Verification items for this drawing (mm, ordinates from the low corner). A direction names the side the tool comes from. Coordinates: 2 decimals unless noted, no trailing zeros. Order: outer loops, then holes, each group sorted by start corner. A loop starts at its lowest first (then second) coordinate and runs counter-clockwise, first axis right, second up. Notation, with made-up numbers: M 46,-6.75 L 80,-6.75 A14 cw 80,19.25 Z; hole C 51,78.25 d7. An arc over 180 degrees is marked long. Write item = value, one per line.
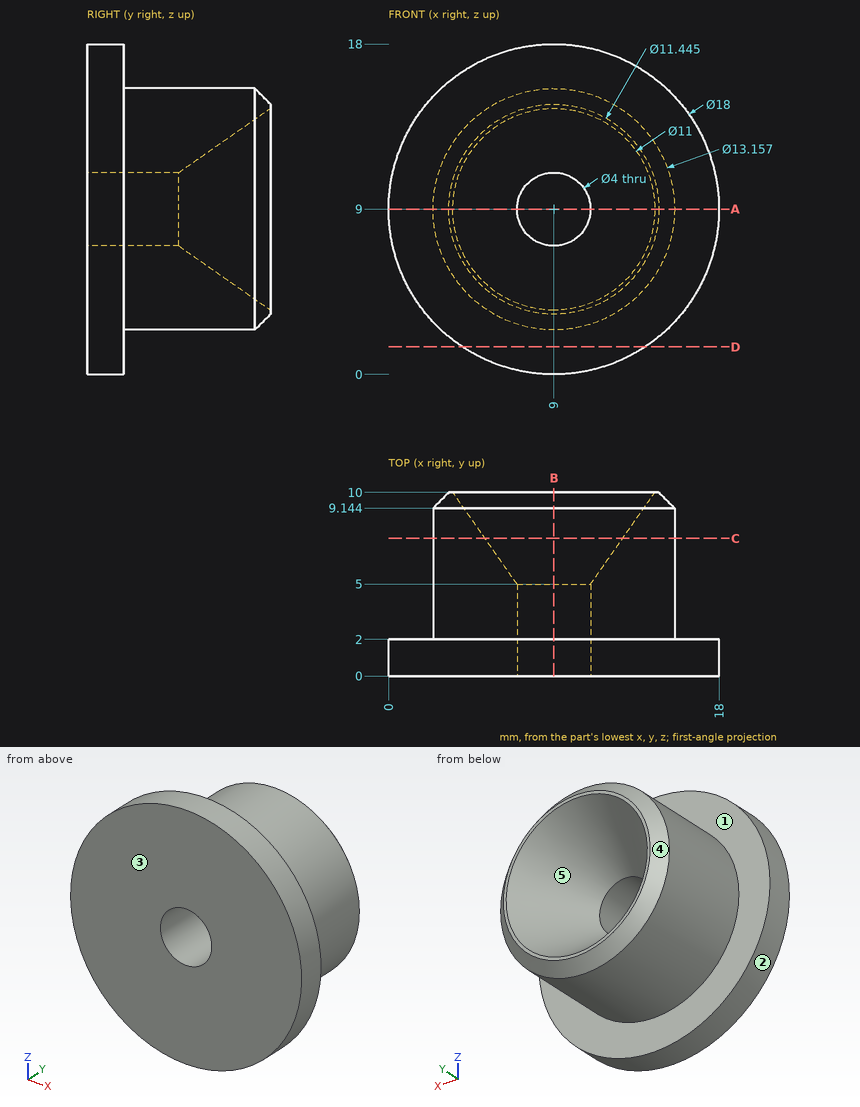
Item 1: Sectioned sample at D-D, the plane z = 1.5. Enter the section's corners in (x, y), then the cut area to 3 significant figures.
Report:
outline = M 4.03,0 L 13.97,0 L 13.97,2 L 4.03,2 Z
area = 19.9 mm^2
Item 2: Sectioned sample at C-C, the plane y = 7.5. Enter the section's corners in (x, z).
Report:
outline = C 9,9 d13.16; hole C 9,9 d7.5
Item 3: Scan lines: L1, parallel to X at y = 3.2, z = 9; L2, parallel to X at y = 1.4, z = 9. Record each from-to range of solid material in increasing order. Write a range as from..to.
Report:
L1 = 2.42..7, 11..15.58
L2 = 0..7, 11..18
Item 4: Release check for a two-part mould opening along Z. For the marked faces 3, 4 and 5 record: pulls with the +Z half, pulls with the -Z half, needs draft (parallel to the pull), parting line crosses it, or undercut.
Report:
face_3 = needs draft
face_4 = parting line crosses it
face_5 = undercut
Item 5: Gauge pin test, flat ends, axial feed: pin 1 (9 mm diameter, centred on x = 7, z = 9.5, fed in from +Y); pin 2 (3 mm diameter, centred on x = 9, y = 8.5, fed in from -Z); pin 3 (3 mm diameter, centred on x = 10, y = 4.5, fed in from +Z); pin 4 (5 mm diameter, centred on x = 4.5, z = 2, fed in from +Y). Record the tip position at first contact, or that the pin passes through.
Report:
pin_1 = 10
pin_2 = 2.42
pin_3 = 15.58
pin_4 = 9.9
Item 6: Tool access check on the marked faces 1 and 2. Record the directions out of +Z, -Z, +X, -X, +Y, -Y that give a thin tool (end or side, any length) a straight path to the whole face; none if there is none.
Report:
face_1 = +Y
face_2 = +Y, -Y
Item 7: Sectioned sample at B-B, the plane x = 9. Enter the section's corners in (y, z).
Report:
outline = M 0,0 L 2,0 L 2,2.42 L 9.14,2.42 L 10,3.28 L 10,3.5 L 5,7 L 0,7 Z; M 0,11 L 5,11 L 10,14.5 L 10,14.72 L 9.14,15.58 L 2,15.58 L 2,18 L 0,18 Z
Item 8: Sectioned sample at A-A, the plane z = 9. Enter the section's corners in (x, y).
Report:
outline = M 0,0 L 7,0 L 7,5 L 3.5,10 L 3.28,10 L 2.42,9.14 L 2.42,2 L 0,2 Z; M 11,0 L 18,0 L 18,2 L 15.58,2 L 15.58,9.14 L 14.72,10 L 14.5,10 L 11,5 Z
